Could you check a few things on this model? Use its own coordinates, in mm. Round coordinates to 2 decimals unless told otherwise and drop trailing zeros. Write each loop counter-clockwise with the first axis right and the second up, starting at its lowest first coordinate (ties: lowest second). Pieces come first, ordered by that corner, then holes. Notation, with made-up numbers: (-7.75, 82) -> (11.25, 82) arc R27 ccw to (11.25, 100) -> close; hole circle Ø2 at (11, -30.75). An arc over 180 degrees is marked (long way). Return JSON: item names as keys, results as strings.
from build123d import *

# Parameters (mm, degrees)
PAD_DEPTH    = 28
SKETCH001_R  = 21.2
POCKET_DEPTH = 24
FILLET_R     = 3
FILLET001_R  = 2
FILLET002_R  = 2


with BuildPart() as part:
    # Sketch (on XY_Plane of Origin) → Pad (new body)
    with BuildSketch(Plane.XY):
        Polygon((21.125697, -17.605536), (27.387118, 2.48913), (17.605536, 21.125697), (-2.48913, 27.387118), (-21.125697, 17.605536), (-27.387118, -2.48913), (-17.605536, -21.125697), (2.48913, -27.387118), align=None)
    extrude(amount=PAD_DEPTH)

    # Sketch001 (on Face10 of Pad) → Pocket (cut)
    with BuildSketch(Plane.XY.offset(28)):
        Circle(SKETCH001_R)
    extrude(amount=-POCKET_DEPTH, mode=Mode.SUBTRACT)

    # Fillet
    fillet_edges = [part.edges().sort_by_distance(p)[0] for p in [
        (2.48913, -27.387118, 14),
        (21.125697, -17.605536, 14),
        (27.387118, 2.48913, 14),
        (17.605536, 21.125697, 14),
        (-2.48913, 27.387118, 14),
        (-21.125697, 17.605536, 14),
        (-27.387118, -2.48913, 14),
        (-17.605536, -21.125697, 14),
    ]]
    fillet(fillet_edges, radius=FILLET_R)

    # Fillet001
    fillet001_edges = [part.edges().sort_by_distance(p)[0] for p in [
        (-24.256408, 7.558203, 0),
        (-11.807414, 22.496327, 0),
        (7.558203, 24.256408, 0),
        (22.496327, 11.807414, 0),
        (24.256408, -7.558203, 0),
        (11.807414, -22.496327, 0),
        (-7.558203, -24.256408, 0),
        (-22.496327, -11.807414, 0),
    ]]
    fillet(fillet001_edges, radius=FILLET001_R)

    # Fillet002
    fillet002_edges = [part.edges().sort_by_distance(p)[0] for p in [
        (22.496327, 11.807414, 28),
        (24.256408, -7.558203, 28),
        (11.807414, -22.496327, 28),
        (7.558203, 24.256408, 28),
        (-11.807414, 22.496327, 28),
        (-24.256408, 7.558203, 28),
        (-22.496327, -11.807414, 28),
        (-7.558203, -24.256408, 28),
    ]]
    fillet(fillet002_edges, radius=FILLET002_R)


solid = part.part
1) I want a section at A-A, the plane z = 13. Please give me the cut outline in (x, y).
Return value:
{"outline": "(-27.02, -1.3) arc R3 ccw to (-26.81, -3.59) -> (-18.18, -20.03) arc R3 ccw to (-16.42, -21.5) -> (1.3, -27.02) arc R3 ccw to (3.59, -26.81) -> (20.03, -18.18) arc R3 ccw to (21.5, -16.42) -> (27.02, 1.3) arc R3 ccw to (26.81, 3.59) -> (18.18, 20.03) arc R3 ccw to (16.42, 21.5) -> (-1.3, 27.02) arc R3 ccw to (-3.59, 26.81) -> (-20.03, 18.18) arc R3 ccw to (-21.5, 16.42) -> close; hole circle Ø42.4 at (0, 0)"}
2) Thinking about a two-plate mould opening in X: for faces 1 (the face through (19.583, -8.12, 16.168)), 2 (the face through (7.68, 24.22, 13.83)), 3 (the face through (-7.26, -23.72, 0.57)), which applies, pulls with the +X half, pulls with the -X half, needs draft (parallel to the pull), parting line crosses it, or undercut?
Return value:
{"face 1": "undercut", "face 2": "pulls with the +X half", "face 3": "pulls with the -X half"}
3) If I drill on probe 1 along Z at (x, y) = (2.5, -11); probe 2 along Y at (x, z) = (-4.5, 13); probe 3 along X at (y, z) = (15, 15.25), over which ranges is the centre line in solid material (lowest first)? Write a range as [from, to].
Return value:
{"probe 1": "[0, 4]", "probe 2": "[-25.21, -20.72], [20.72, 26.33]", "probe 3": "[-21.94, -14.98], [14.98, 20.82]"}
4) Will these pins go through, and if not, where does the flat tip stop? pin 1 Ø12 at (y, z) = (11, 8.5) entering from -X; pin 2 Ø21 at (x, y) = (-5.5, -8) entering from +Z; pin 3 Ø3 at (y, z) = (-8, 7.5) entering from -X; pin 4 Ø6 at (y, z) = (-0.5, 18.5) entering from +X.
Return value:
{"pin 1": "x = -25.05", "pin 2": "z = 4", "pin 3": "x = -25.28", "pin 4": "x = 27.15"}
